Could you check a few things on this drawing? It's one solid part, dimensions in mm from its lowest x, y, z. A direction names the side the tool comes from. Give positions to 0.01 mm unless a question says otherwise; leave off trailing zeros. Loops run counter-clockwise (first coordinate to the right, second up) from the corner with the lowest first, then second, coordinate; pieces in that order, holes last.
Q1. I need wall thicknesses on probe 1 along Y at (x, z) = (30.2, 9.5); probe 2 along Y at (x, z) = (12.5, 6.5); probe 3 along X at (y, z) = (61, 5). Which ranges of each line are inside material? Lowest first, please.
Q2. Suppose I cut it at C-C (z = 10). List the corners of the cut face in (x, y) for me.
Q3. Suppose I cut it at D-D (y = 68.5). List the corners of the cut face in (x, z) for me, and give its area (3 significant figures).
Q4. Thinking about a two-plate mould opening in Y: for the marked faces 4, 5 and 6, which applies, pulls with the +Y half, pulls with the -Y half, needs draft (parallel to the pull), parting line crosses it, or undercut?
Q5. Suppose I cut it at A-A (x = 75.2). List the corners of the cut face in (y, z) for me.
Q6. For the marked faces 1, 2 and 3, which set-ups out of +Z, -Z, +X, -X, +Y, -Y let a thin tool reach every point of the face, with its end or its side?
Q7. Suppose I cut it at B-B (x = 19). List the corners of the cut face in (y, z) for me.
Q8. I'm going to push flat-ended pins straight in: P1, Ø1.5, axis at y = 131, z = 3, coming from the +X side; P2, Ø6, axis at x = 30.2, y = 102.01, coming from the -Z side; P3, Ø2, axis at y = 103.5, z = 6.5, coming from the -X side. Where does each tip first touch, or does it pass through?
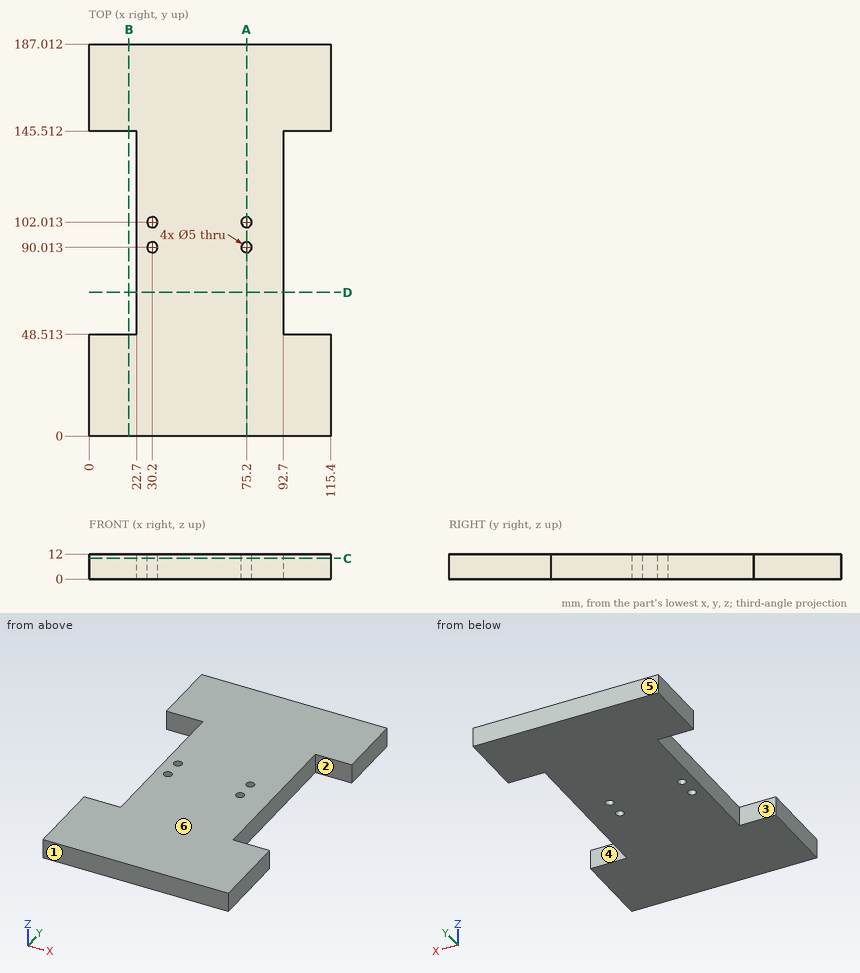
Solutions:
1. probe 1: y = 0 to 87.51, 92.51 to 99.51, 104.51 to 187.01
1. probe 2: y = 0 to 48.51, 145.51 to 187.01
1. probe 3: x = 22.7 to 92.7
2. outline: (0, 0) - (115.4, 0) - (115.4, 48.51) - (92.7, 48.51) - (92.7, 145.51) - (115.4, 145.51) - (115.4, 187.01) - (0, 187.01) - (0, 145.51) - (22.7, 145.51) - (22.7, 48.51) - (0, 48.51) - close; hole circle Ø5 at (30.2, 90.01); hole circle Ø5 at (30.2, 102.01); hole circle Ø5 at (75.2, 90.01); hole circle Ø5 at (75.2, 102.01)
3. outline: (22.7, 0) - (92.7, 0) - (92.7, 12) - (22.7, 12) - close
3. area: 840 mm2
4. face 4: undercut
4. face 5: pulls with the +Y half
4. face 6: needs draft
5. outline: (0, 0) - (87.51, 0) - (87.51, 12) - (0, 12) - close; (92.51, 0) - (99.51, 0) - (99.51, 12) - (92.51, 12) - close; (104.51, 0) - (187.01, 0) - (187.01, 12) - (104.51, 12) - close
6. face 1: +Z, -Z, +X, -X, -Y
6. face 2: +Z, -Z, +X
6. face 3: +Z, -Z, -X
7. outline: (0, 0) - (48.51, 0) - (48.51, 12) - (0, 12) - close; (145.51, 0) - (187.01, 0) - (187.01, 12) - (145.51, 12) - close
8. P1: stops at x = 92.7
8. P2: stops at z = 0
8. P3: stops at x = 22.7
